The listing builds one solid part. Answer for the finished solid, in the listing's coordinates (mm). A direction names the side the tool comes from. Round coordinates to 2 decimals unless told otherwise and drop trailing zeros. Order: outer loops, then holes, each group sorted by start corner. A loop starts at its lowest first (then second) coordinate and runs counter-clockwise, first axis right, second up. Notation, with made-up numbers: (26.25, -30.75) -> (70.25, -30.75) arc R31 cw to (70.25, 5.25) -> close; hole circle Ø6 at (57.5, -21.75). An arc over 180 degrees is marked (long way). Return JSON: item names as keys, results as strings. Group by question number.
(1) Determine the mould class of faces 4 (the face through (72, 299.382, 3)), 5 (the face through (87, 57.232, 3)), 6 (the face through (81.772, 69.32, 2.958)), 7 (the face through (49, 299.382, 3)) for opening direction X: +X half, -X half, draft (parallel to the pull), parting line (faces both ways), or undercut.
(2) Which of the six approach directions +Z, -Z, +X, -X, +Y, -Y give full straight-line access (tool end or side, diameter ignored) to faces 1 (the face through (61, 6.232, 3)), 2 (the face through (54.919, 200, 3)), 3 (the face through (81.771, 47, 3))?
(3) Consider line 1 (Y direction, x = 87.5, z = 4.9); line 2 (Y direction, x = 75, z = 2.95); line 3 (Y direction, x = 64.5, z = 5.4). Determine where each line is inside the solid, lowest interval first. Write a range as [from, to].
(4) Each of these flat-tipped pins is pushed along its axis until it touches: pin 1 (1.8 mm diameter, centred on y = 44, z = 2, fed in from +X); pin 2 (3 mm diameter, centred on x = 46.77, y = 234.58, fed in from +Z). Where does it stop, or does it pass through?
(5) The part is cut by section B-B (z = 4.45). Count the separate pieces of the cut face and the enclosed holes in it, plus the area to 3 significant figures.
(6) The part is cut by section A-A (y = 161.5). Determine the outline of the cut face in (x, z), plus the area to 3 significant figures.
from build123d import *

# Parameters (mm, degrees)
MODEL_R                  = 1.8
MODEL_W                  = 9.199995837
MODEL_H                  = 6.900001917
MODEL_W_2                = 9.1999977
MODEL_W_3                = 15.39999384
MODEL_H_2                = 6.899997952
MODEL_W_4                = 6.900001918
MODEL_H_3                = 9.199995837
MODEL_H_4                = 9.1999977
MODEL_H_5                = 9.199997699
RESSALTO_EXTRUS_O1_DEPTH = 6


with BuildPart() as part:
    # Model → Ressalto-extrusão1 (new body)
    with BuildSketch(Plane.XY):
        with BuildLine():
            Line((89.771252514, 6.232071499), (31.271271234, 6.232071499))
            Line((31.271271234, 6.232071499), (31.271271234, 302.231976779))
            Line((31.271271234, 302.231976779), (89.771252514, 302.231976779))
            Line((89.771252514, 302.231976779), (89.771252514, 271.231986699))
            Line((89.771252514, 271.231986699), (83.771254434, 271.231986699))
            Line((83.771254434, 271.231986699), (81.771255074, 269.231987339))
            Line((81.771255074, 269.231987339), (81.771255074, 253.231992459))
            Line((81.771255074, 253.231992459), (83.771254434, 251.231993099))
            Line((83.771254434, 251.231993099), (89.771252514, 251.231993099))
            Line((89.771252514, 251.231993099), (89.771252514, 243.231995659))
            Line((89.771252514, 243.231995659), (85.771253794, 243.231995659))
            ThreePointArc((85.771253794, 243.231995659), (81.771255074, 239.231996939), (85.771253794, 235.231998219))
            Line((85.771253794, 235.231998219), (89.771252514, 235.231998219))
            Line((89.771252514, 235.231998219), (89.771252514, 157.982022859))
            Line((89.771252514, 157.982022859), (83.771254434, 157.982022859))
            Line((83.771254434, 157.982022859), (81.771255074, 155.982023499))
            Line((81.771255074, 155.982023499), (81.771255074, 152.482024779))
            Line((81.771255074, 152.482024779), (83.771254434, 150.482025419))
            Line((83.771254434, 150.482025419), (89.771252514, 150.482025419))
            Line((89.771252514, 150.482025419), (89.771252514, 73.232050059))
            Line((89.771252514, 73.232050059), (85.771253794, 73.232050059))
            ThreePointArc((85.771253794, 73.232050059), (81.771255074, 69.232051339), (85.771253794, 65.232052619))
            Line((85.771253794, 65.232052619), (89.771252514, 65.232052619))
            Line((89.771252514, 65.232052619), (89.771252514, 57.232055179))
            Line((89.771252514, 57.232055179), (83.771254434, 57.232055179))
            Line((83.771254434, 57.232055179), (81.771255074, 55.232055819))
            Line((81.771255074, 55.232055819), (81.771255074, 39.232060939))
            Line((81.771255074, 39.232060939), (83.771254434, 37.232061579))
            Line((83.771254434, 37.232061579), (89.771252514, 37.232061579))
            Line((89.771252514, 37.232061579), (89.771252514, 6.232071499))
        make_face()
        with Locations((60.621261842, 12.532070537)):
            Circle(MODEL_R, mode=Mode.SUBTRACT)
        with Locations((83.771254434, 61.233170309)):
            Circle(MODEL_R, mode=Mode.SUBTRACT)
        with Locations((77.271256514, 69.232051339)):
            Circle(MODEL_R, mode=Mode.SUBTRACT)
        with Locations((83.771254434, 77.232048779)):
            Circle(MODEL_R, mode=Mode.SUBTRACT)
        with Locations((46.771271234, 73.882024139)):
            Circle(MODEL_R, mode=Mode.SUBTRACT)
        with Locations((37.571269218, 107.832043016)):
            Circle(MODEL_R, mode=Mode.SUBTRACT)
        with Locations((37.571269218, 200.632005262)):
            Circle(MODEL_R, mode=Mode.SUBTRACT)
        with Locations((46.771271234, 234.582024139)):
            Circle(MODEL_R, mode=Mode.SUBTRACT)
        with Locations((83.771254434, 231.233115909)):
            Circle(MODEL_R, mode=Mode.SUBTRACT)
        with Locations((77.271256514, 239.231996939)):
            Circle(MODEL_R, mode=Mode.SUBTRACT)
        with Locations((83.771254434, 247.231994379)):
            Circle(MODEL_R, mode=Mode.SUBTRACT)
        with Locations((60.521261874, 295.931975819)):
            Circle(MODEL_R, mode=Mode.SUBTRACT)
        with Locations((72.521257893, 12.532071498)):
            Rectangle(MODEL_W, MODEL_H, mode=Mode.SUBTRACT)
        with Locations((48.621267095, 295.931976781)):
            Rectangle(MODEL_W_2, MODEL_H, mode=Mode.SUBTRACT)
        with Locations((64.371263002, 147.032026443)):
            Rectangle(MODEL_W_3, MODEL_H_2, mode=Mode.SUBTRACT)
        with Locations((37.571270179, 95.932046966)):
            Rectangle(MODEL_W_4, MODEL_H_3, mode=Mode.SUBTRACT)
        with Locations((72.421257924, 295.931976781)):
            Rectangle(MODEL_W, MODEL_H, mode=Mode.SUBTRACT)
        with Locations((37.571270179, 212.532000041)):
            Rectangle(MODEL_W_4, MODEL_H_4, mode=Mode.SUBTRACT)
        with Locations((37.571270179, 119.732037796)):
            Rectangle(MODEL_W_4, MODEL_H_5, mode=Mode.SUBTRACT)
        with Locations((48.721267063, 12.532071498)):
            Rectangle(MODEL_W_2, MODEL_H, mode=Mode.SUBTRACT)
        with Locations((37.571270179, 188.732009212)):
            Rectangle(MODEL_W_4, MODEL_H_3, mode=Mode.SUBTRACT)
        with Locations((64.371263002, 161.432021835)):
            Rectangle(MODEL_W_3, MODEL_H_2, mode=Mode.SUBTRACT)
        Polygon((54.919245732, 207.685602791), (52.679245732, 210.065602791), (48.199248599, 210.065602791), (45.959248599, 207.685602791), (45.959248599, 193.410404919), (48.199248599, 191.030404919), (52.679245732, 191.030404919), (54.919245732, 193.410404919), align=None, mode=Mode.SUBTRACT)
    extrude(amount=RESSALTO_EXTRUS_O1_DEPTH)


solid = part.part
Answer below:
{
 "1": {"face 4": "undercut", "face 5": "draft", "face 6": "+X half", "face 7": "undercut"},
 "2": {"face 1": "+Z, -Z, +X, -X, -Y", "face 2": "+Z, -Z", "face 3": "+Z, -Z, +X"},
 "3": {"line 1": "y = [6.23, 37.23], [57.23, 65.23], [73.23, 150.48], [157.98, 235.23], [243.23, 251.23], [271.23, 302.23]", "line 2": "y = [6.23, 9.08], [15.98, 292.48], [299.38, 302.23]", "line 3": "y = [6.23, 143.58], [150.48, 157.98], [164.88, 302.23]"},
 "4": {"pin 1": "stops at x = 81.77", "pin 2": "passes through"},
 "5": {"separate pieces": "1", "enclosed holes": "23", "area": "15,800 mm²"},
 "6": {"outline": "(31.27, 0) -> (56.67, 0) -> (56.67, 6) -> (31.27, 6) -> close; (72.07, 0) -> (89.77, 0) -> (89.77, 6) -> (72.07, 6) -> close", "area": "259 mm²"}
}
